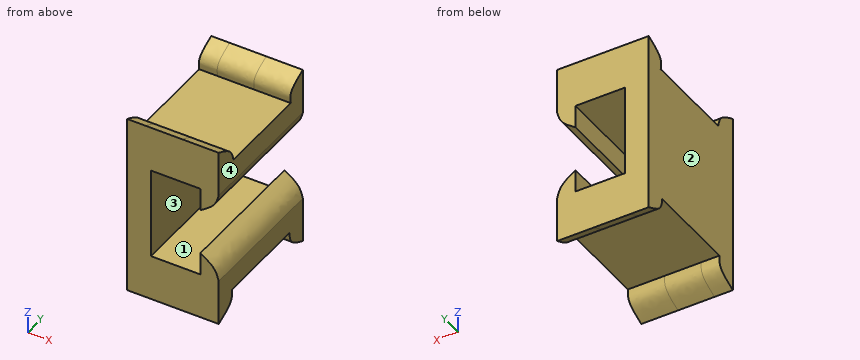
```python
from build123d import *

# Parameters (mm, degrees)
F1_DEPTH  = 5.08
F2_W      = 9.398
F2_H      = 12.7
F3_DEPTH  = 36.4129
F5_W      = 19.05
F5_H      = 3.175
F4_W      = 19.05
F4_H      = 3.175
F6_DEPTH  = 2.54
F8_DEPTH  = 25.4
F10_DEPTH = 2.54


with BuildPart() as f1:
    # F0 (on Right) → F1 (new body, symmetric)
    with BuildSketch(Plane.YZ):
        Polygon((-9.525, 42.7627552986), (-9.525, 23.7127552986), (-6.4988480881, 23.7127552986), (6.468560081, 23.7127552986), (9.525, 23.7127552986), (9.525, 42.7627552986), (6.8012457341, 42.7627552986), (-6.1935493723, 42.7627552986), align=None)
        with BuildLine():
            Line((-9.525, 45.9377552986), (-9.525, 42.7627552986))
            Line((-9.525, 42.7627552986), (-6.1935493723, 42.7627552986))
            add(Edge.make_bspline(
                [(-9.525, 45.9377552986), (-8.4843289073, 45.4587623907), (-6.6623733691, 44.6201652706), (-6.3342528413, 43.3202012234), (-6.1935493723, 42.7627552986)],
                knots=[0, 0, 0, 0, 0.5711835832, 1, 1, 1, 1], degree=3))
        make_face()
        with BuildLine():
            add(Edge.make_bspline(
                [(9.525, 45.9377552986), (8.4082384885, 45.4684357534), (6.487493932, 44.6612419592), (6.708667258, 43.3229401352), (6.8012457341, 42.7627552986)],
                knots=[0, 0, 0, 0, 0.5814211514, 1, 1, 1, 1], degree=3))
            Line((6.8012457341, 42.7627552986), (9.525, 42.7627552986))
            Line((9.525, 42.7627552986), (9.525, 45.9377552986))
        make_face()
        with BuildLine():
            Line((-6.4988480881, 23.7127552986), (-9.525, 23.7127552986))
            Line((-9.525, 23.7127552986), (-9.525, 20.5377552986))
            add(Edge.make_bspline(
                [(-9.525, 20.5377552986), (-8.3782583984, 21.004520321), (-6.4146620617, 21.8037745617), (-6.4741154988, 23.1519254498), (-6.4988480881, 23.7127552986)],
                knots=[0, 0, 0, 0, 0.5840006829, 1, 1, 1, 1], degree=3))
        make_face()
        with BuildLine():
            Line((9.525, 23.7127552986), (6.468560081, 23.7127552986))
            add(Edge.make_bspline(
                [(9.525, 20.5377552986), (8.483129389, 21.0137326336), (6.6694729366, 21.8422994016), (6.528535002, 23.1544015571), (6.468560081, 23.7127552986)],
                knots=[0, 0, 0, 0, 0.5744586355, 1, 1, 1, 1], degree=3))
            Line((9.525, 20.5377552986), (9.525, 23.7127552986))
        make_face()
    extrude(amount=F1_DEPTH, both=True)

    # F2 (on face) → F3 (cut)
    with BuildSketch(Plane.XZ.offset(9.525)):
        with Locations((0.381, 33.2377552986)):
            Rectangle(F2_W, F2_H)
    extrude(amount=-F3_DEPTH, mode=Mode.SUBTRACT)

    # F5 (on face) + F4 (on face) → F6 (join)
    with BuildSketch(Plane.YZ.offset(5.08)):
        with Locations((0, 28.4752552986)):
            Rectangle(F5_W, F5_H)
    with BuildSketch(Plane.YZ.offset(5.08)):
        with Locations((0, 38.0002552986)):
            Rectangle(F4_W, F4_H)
    extrude(amount=-F6_DEPTH)

    # F7 (on face) → F8 (cut)
    with BuildSketch(Plane.XZ.offset(9.525)):
        with BuildLine():
            Line((5.08, 36.4127552986), (5.08, 39.5877552986))
            add(Edge.make_bspline(
                [(5.08, 39.5877552986), (4.9399237186, 39.0382267482), (4.6311542423, 37.8269035964), (3.2788294654, 36.9123905765), (2.54, 36.4127552986)],
                knots=[0, 0, 0, 0, 0.4536597435, 1, 1, 1, 1], degree=3))
            Line((2.54, 36.4127552986), (5.08, 36.4127552986))
        make_face()
        with BuildLine():
            add(Edge.make_bspline(
                [(5.08, 26.8877552986), (4.9399237186, 27.437283849), (4.6311542423, 28.6486070008), (3.2788294654, 29.5631200208), (2.54, 30.0627552986)],
                knots=[0, 0, 0, 0, 0.4536597435, 1, 1, 1, 1], degree=3))
            Line((5.08, 26.8877552986), (5.08, 30.0627552986))
            Line((5.08, 30.0627552986), (2.54, 30.0627552986))
        make_face()
    extrude(amount=-F8_DEPTH, mode=Mode.SUBTRACT)

    # F9 (on face) → F10 (join)
    with BuildSketch(Plane(origin=(-5.08, 0, 0), x_dir=(0, -1, 0), z_dir=(-1, 0, 0))):
        with BuildLine():
            add(Edge.make_bspline(
                [(-9.525, 20.5377552986), (-8.483129389, 21.0137326336), (-6.6694729366, 21.8422994016), (-6.528535002, 23.1544015571), (-6.468560081, 23.7127552986)],
                knots=[0, 0, 0, 0, 0.5744586355, 1, 1, 1, 1], degree=3))
            Line((-6.468560081, 23.7127552986), (6.4988480881, 23.7127552986))
            add(Edge.make_bspline(
                [(9.525, 20.5377552986), (8.3782583984, 21.004520321), (6.4146620617, 21.8037745617), (6.4741154988, 23.1519254498), (6.4988480881, 23.7127552986)],
                knots=[0, 0, 0, 0, 0.5840006829, 1, 1, 1, 1], degree=3))
            Line((9.525, 20.5377552986), (9.525, 45.9377552986))
            add(Edge.make_bspline(
                [(9.525, 45.9377552986), (8.4843289073, 45.4587623907), (6.6623733691, 44.6201652706), (6.3342528413, 43.3202012234), (6.1935493723, 42.7627552986)],
                knots=[0, 0, 0, 0, 0.5711835832, 1, 1, 1, 1], degree=3))
            Line((6.1935493723, 42.7627552986), (-6.8012457341, 42.7627552986))
            add(Edge.make_bspline(
                [(-9.525, 45.9377552986), (-8.4082384885, 45.4684357534), (-6.487493932, 44.6612419592), (-6.708667258, 43.3229401352), (-6.8012457341, 42.7627552986)],
                knots=[0, 0, 0, 0, 0.5814211514, 1, 1, 1, 1], degree=3))
            Line((-9.525, 45.9377552986), (-9.525, 20.5377552986))
        make_face()
    extrude(amount=F10_DEPTH)


solid = f1.part
```
For this review, take the finished solid that the model builds, in its own axes (mm). Face numbers are marked on the shaded views. A direction names the side the tool comes from. Give positions to 0.01 mm unless a question says otherwise; leave off trailing zeros. Write each loop counter-clockwise with the first axis right and the second up, starting at its lowest first coordinate (ties: lowest second). Pieces come first, ordered by that corner, then holes. Notation, with made-up numbers: M 86.5,83.25 L 111.5,83.25 A22 cw 111.5,89.25 Z; hole C 54.5,-19.75 d2. An arc over 180 degrees is marked long. Answer as CSV lines item,"result".
1. Draft analysis for pull direction Z (two halves, no side actions). For the marked faces 3 and 4, state which applies: +Z half, -Z half, draft (parallel to the pull), parting line (faces both ways), or undercut.
Findings:
face 3,"undercut"
face 4,"draft"
2. For pin 1 (1 mm diameter, centred on x = -2.5, y = 7, fed in from +Z); pin 2 (3 mm diameter, centred on x = 3, y = 3, fed in from -Z); pin 3 (3.5 mm diameter, centred on x = -1.5, y = 4, fed in from +Z), all flat-tipped, find the tip position at first contact; note any pin that passes through.
Findings:
pin 1,"stops at z = 44.94"
pin 2,"stops at z = 23.71"
pin 3,"stops at z = 42.76"
3. Wall thickness on line 1 (Z direction, x = -1.75, y = 3); line 2 (X direction, y = -7.5, z = 29.5); line 3 (X direction, y = -2, z = 28.75): over which ranges is each line inside the solid? List them lowest first.
Findings:
line 1,"z = 23.71 to 26.89, 39.59 to 42.76"
line 2,"x = -7.62 to -4.32, 2.54 to 3.35"
line 3,"x = -7.62 to -4.32, 2.54 to 4.22"
4. Consider section A-A, the plane z = 33. Write out the cut boundary in (x, y) (3 decimals), then the cut area to 3 significant figures.
Findings:
outline,"M -7.62,-9.525 L -4.318,-9.525 L -4.318,9.525 L -7.62,9.525 Z"
area,"62.9 mm2"
5. For the marked faces 1 and 2, list the 3-axis set-ups (+Z, -Z, +X, -X, +Y, -Y) from which the entire face can be reached by the end or side of a thin tool; tool diameter is ignored.
Findings:
face 1,"+Y, -Y"
face 2,"+Z, -Z, -X, +Y, -Y"
